from build123d import *

# Parameters (mm, degrees)
BOSS_EXTRUDE1_DEPTH = 6.1
SKETCH3_R           = 18.340849868
SKETCH3_R_2         = 10.340849868
BOSS_EXTRUDE2_DEPTH = 6.2


with BuildPart() as part:
    # Sketch2 → Boss-Extrude1 (new body)
    with BuildSketch(Plane.XY):
        Polygon((9.301598931, 56.02003156), (-4.198401069, 56.02003156), (-4.198401069, 48.443721), (-4.198401069, -16.02003156), (-3.039250937, -16.02003156), (-3.039250937, -56.02003156), (4.960749063, -56.02003156), (4.960749063, -20.437234175), (9.301598931, -20.437234175), (9.301598931, 48.443721), align=None)
        Polygon((-4.198401069, 49.063721), (-4.198401069, 53.74676634), (-9.301598931, 52.089011931), (-9.301598931, 50.721475409), align=None)
        Polygon((-4.198401069, 43.76067566), (-4.198401069, 48.443721), (-9.301598931, 46.785966591), (-9.301598931, 45.418430069), align=None)
        Polygon((-4.198401069, 38.46067566), (-4.198401069, 43.143721), (-9.301598931, 41.485966591), (-9.301598931, 40.118430069), align=None)
        Polygon((-4.198401069, 33.16067566), (-4.198401069, 37.843721), (-9.301598931, 36.185966591), (-9.301598931, 34.818430069), align=None)
        Polygon((-4.198401069, 27.86067566), (-4.198401069, 32.543721), (-9.301598931, 30.885966591), (-9.301598931, 29.518430069), align=None)
        Polygon((-9.301598931, 24.218430069), (-4.198401069, 22.56067566), (-4.198401069, 27.243721), (-9.301598931, 25.585966591), align=None)
        Polygon((-9.301598931, 18.918430069), (-4.198401069, 17.26067566), (-4.198401069, 21.943721), (-9.301598931, 20.285966591), align=None)
        Polygon((-9.301598931, 13.618430069), (-4.198401069, 11.96067566), (-4.198401069, 16.643721), (-9.301598931, 14.985966591), align=None)
    extrude(amount=BOSS_EXTRUDE1_DEPTH)

    # Sketch3 → Boss-Extrude2 (add)
    with BuildSketch(Plane.XZ.offset(56.02003156)):
        with Locations(Location((15.301598931, 2.942643244, 0), (0, 0, 170.087216978))):
            Circle(SKETCH3_R)
        with Locations(Location((15.301598931, 2.942643244, 0), (0, 0, 180))):
            Circle(SKETCH3_R_2, mode=Mode.SUBTRACT)
    extrude(amount=BOSS_EXTRUDE2_DEPTH)


solid = part.part
Work out the finished part from the listing and answer in its coordinate system (mm). A direction names the side the tool comes from. Coordinates: 2 decimals unless noted, no trailing zeros. Write each loop counter-clockwise with the first axis right and the second up, starting at its lowest first coordinate (ties: lowest second). Pieces come first, ordered by that corner, then holes. Notation, with made-up numbers: M 29,61 L 56,61 A28 ccw 56,92 Z; hole C 42,34 d10. An arc over 180 degrees is marked long. Use one line per item in the form item = value. Start each with the question number.
1. The part is cut by section B-B (z = 10). Give the vertices of the cut face in (x, y).
2. The part is cut by section A-A (x = 11). Give the vertices of the cut face in (y, z), plus the area to 3 significant figures.
3. A tool of negligible diameter and unlimited length cuts with its end or side. For faces 1 (the face through (-6.786, 23.401, 3.007)), 2 (the face through (-3.039, -36, 3)), 3 (the face through (-4.198, 55, 3)), from which of +Z, -Z, +X, -X, +Y, -Y can it reach the whole face along a straight path? Write none if from no direction.
4. Straight lines are drawn through the part: probe 1 along Y at (x, z) = (25, 14); probe 2 along Z at (x, y) = (2, 39); probe 3 along X at (y, z) = (-43.5, 1.5). For each, find the intervals that lie inside material, in ascending order. Write a range as from..to.
5. The part is cut by section D-D (z = 18.5). Give the vertices of the cut face in (x, y), plus the area to 3 significant figures.
6. Each of these flat-tipped pins is pushed along its axis until it touches: P1, Ø3, axis at x = -4.5, y = 2, coming from the +Z side; P2, Ø0.6, axis at x = -3.5, z = 3.5, coming from the -Y side; P3, Ø3, axis at y = 26, z = 8.5, coming from the +X side; P4, Ø6.5, axis at y = 0, z = 3.5, coming from the +X side. Where does it stop, or does it pass through?
7. The part is cut by section C-C (y = 1). Give the vertices of the cut face in (x, z).
Evaluation:
q1.outline = M -1.63,-62.22 L 7.74,-62.22 L 7.74,-56.02 L -1.63,-56.02 Z; M 22.86,-62.22 L 32.23,-62.22 L 32.23,-56.02 L 22.86,-56.02 Z
q2.outline = M -62.22,-14.89 L -56.02,-14.89 L -56.02,-6.46 L -62.22,-6.46 Z; M -62.22,12.35 L -56.02,12.35 L -56.02,20.77 L -62.22,20.77 Z
q2.area = 104 mm^2
q3.face_1 = +Z, -Z, -X
q3.face_2 = +Z, -Z, -X, -Y
q3.face_3 = +Z, -Z, -X, +Y
q4.probe_1 = -62.22..-56.02
q4.probe_2 = 0..6.1
q4.probe_3 = -3.04..4.96
q5.outline = M 5.59,-62.22 L 25.02,-62.22 L 25.02,-56.02 L 5.59,-56.02 Z
q5.area = 120 mm^2
q6.P1 = 6.1
q6.P2 = -16.02
q6.P3 = through
q6.P4 = 9.3
q7.outline = M -4.2,0 L 9.3,0 L 9.3,6.1 L -4.2,6.1 Z
